Can you work these out from the model? Positions are in its coordinate system, mm. A direction names the side the tool comes from. Round coordinates to 2 decimals unless told otherwise and drop trailing zeros. Loops run counter-clockwise (first coordinate to the right, second up) from the corner with the lowest first, then second, coordinate; pieces in that order, holes last. Notation, with made-up numbers: (-12.5, 77) - (3.5, 77) arc R27 ccw to (3.5, 94) - close; hole circle Ø10 at (-15, -30). An arc over 180 degrees is marked (long way). Answer as CSV lines item,"result".
```python
from build123d import *

# Parameters (mm, degrees)
SKETCH_1_W          = 28.5
SKETCH_1_H          = 28.5
SKETCH_1_W_2        = 24.5
SKETCH_1_H_2        = 24.5
EXTRUDE_1_DEPTH     = 4
CUT_EXTRUDE_1_REACH = 34.114
SKETCH_2_W          = 15
SKETCH_2_H          = 4
EXTRUDE_2_DEPTH     = 1
SKETCH_4_W          = 2
SKETCH_4_H          = 5
EXTRUDE_3_DEPTH     = 7
EXTRUDE_7_DEPTH     = 5
SKETCH_6_W          = 6.5
SKETCH_6_H          = 6
SKETCH_6_R          = 1.75
EXTRUDE_6_DEPTH     = 2
FILLET_1_R          = 2
SKETCH_8_W          = 3
SKETCH_8_H          = 7.25
CUT_EXTRUDE_3_DEPTH = 40.358131307
FILLET_2_R          = 1


with BuildPart() as part:
    # ｽｹｯﾁ1 → ﾎﾞｽ - 押し出し1 (new body)
    with BuildSketch(Plane.XY):
        Rectangle(SKETCH_1_W, SKETCH_1_H)
        Rectangle(SKETCH_1_W_2, SKETCH_1_H_2, mode=Mode.SUBTRACT)
    extrude(amount=EXTRUDE_1_DEPTH)

    # ｽｹｯﾁ2 → ｶｯﾄ - 押し出し1 (cut, up to next)
    with BuildSketch(Plane(origin=(0, -14.25, 0), x_dir=(-1, 0, 0), z_dir=(0, -1, 0)), mode=Mode.PRIVATE) as cut_extrude_1_sk1:
        with Locations((0, -2)):
            Rectangle(SKETCH_2_W, SKETCH_2_H)
    cut_extrude_1_tool1 = extrude(cut_extrude_1_sk1.sketch, amount=-CUT_EXTRUDE_1_REACH, mode=Mode.PRIVATE) & part.part
    add(cut_extrude_1_tool1.solids().sort_by_distance((0, -14.25, 2))[0], mode=Mode.SUBTRACT)

    # ｽｹｯﾁ3 → ﾎﾞｽ - 押し出し2 (add)
    with BuildSketch(Plane(origin=(0, 0, 0), x_dir=(-1, 0, 0), z_dir=(0, 0, -1))):
        Polygon((12.25, 12.25), (12.25, -12.25), (7.5, -12.25), (7.5, -14.25), (14.25, -14.25), (14.25, 14.25), (-14.25, 14.25), (-14.25, -14.25), (-7.5, -14.25), (-7.5, -12.25), (-12.25, -12.25), (-12.25, 12.25), align=None)
        with BuildLine():
            Line((12.25, -12.25), (12.25, -10.25))
            ThreePointArc((12.25, -10.25), (11.664213562, -11.664213562), (10.25, -12.25))
            Line((10.25, -12.25), (12.25, -12.25))
        make_face()
        with BuildLine():
            Line((-7.5, -12.25), (-7.5, -11.25))
            Line((-7.5, -11.25), (-10.25, -11.25))
            ThreePointArc((-10.25, -11.25), (-10.957106781, -10.957106781), (-11.25, -10.25))
            Line((-11.25, -10.25), (-11.25, 10.25))
            ThreePointArc((-11.25, 10.25), (-10.957106781, 10.957106781), (-10.25, 11.25))
            Line((-10.25, 11.25), (10.25, 11.25))
            ThreePointArc((10.25, 11.25), (10.957106781, 10.957106781), (11.25, 10.25))
            Line((11.25, 10.25), (11.25, -10.25))
            ThreePointArc((11.25, -10.25), (10.957106781, -10.957106781), (10.25, -11.25))
            Line((10.25, -11.25), (7.5, -11.25))
            Line((7.5, -11.25), (7.5, -12.25))
            Line((7.5, -12.25), (10.25, -12.25))
            ThreePointArc((10.25, -12.25), (11.664213562, -11.664213562), (12.25, -10.25))
            Line((12.25, -10.25), (12.25, 10.25))
            ThreePointArc((12.25, 10.25), (11.664213562, 11.664213562), (10.25, 12.25))
            Line((10.25, 12.25), (-10.25, 12.25))
            ThreePointArc((-10.25, 12.25), (-11.664213562, 11.664213562), (-12.25, 10.25))
            Line((-12.25, 10.25), (-12.25, -10.25))
            ThreePointArc((-12.25, -10.25), (-11.664213562, -11.664213562), (-10.25, -12.25))
            Line((-10.25, -12.25), (-7.5, -12.25))
        make_face()
        with BuildLine():
            Line((-12.25, -12.25), (-10.25, -12.25))
            ThreePointArc((-10.25, -12.25), (-11.664213562, -11.664213562), (-12.25, -10.25))
            Line((-12.25, -10.25), (-12.25, -12.25))
        make_face()
        with BuildLine():
            Line((-12.25, 12.25), (-12.25, 10.25))
            ThreePointArc((-12.25, 10.25), (-11.664213562, 11.664213562), (-10.25, 12.25))
            Line((-10.25, 12.25), (-12.25, 12.25))
        make_face()
        with BuildLine():
            Line((12.25, 12.25), (10.25, 12.25))
            ThreePointArc((10.25, 12.25), (11.664213562, 11.664213562), (12.25, 10.25))
            Line((12.25, 10.25), (12.25, 12.25))
        make_face()
    extrude(amount=EXTRUDE_2_DEPTH)

    # ｽｹｯﾁ4 → ﾎﾞｽ - 押し出し3 (add)
    with BuildSketch(Plane.XY.offset(4)):
        with Locations((13.25, -2.5)):
            Rectangle(SKETCH_4_W, SKETCH_4_H)
        with Locations((-13.25, -2.5)):
            Rectangle(SKETCH_4_W, SKETCH_4_H)
    extrude(amount=EXTRUDE_3_DEPTH)

    # ｽｹｯﾁ5 → ﾎﾞｽ - 押し出し7 (add)
    with BuildSketch(Plane(origin=(0, 0, 0), x_dir=(1, 0, 0), z_dir=(0, 1, 0))):
        Polygon((12.25, -11), (11.5, -10), (12.25, -10), align=None)
        Polygon((-12.25, -11), (-11.5, -10), (-12.25, -10), align=None)
    extrude(amount=-EXTRUDE_7_DEPTH)

    # ｽｹｯﾁ6 → ﾎﾞｽ - 押し出し6 (add)
    # profile 1 of 2: a face of its own
    with BuildSketch(Plane(origin=(0, 0, -1), x_dir=(-1, 0, 0), z_dir=(0, 0, -1))):
        with Locations((17.5, -3)):
            Rectangle(SKETCH_6_W, SKETCH_6_H)
        with Locations((17.5, -3)):
            Circle(SKETCH_6_R, mode=Mode.SUBTRACT)
    # profile 2 of 2: a face of its own
    with BuildSketch(Plane(origin=(0, 0, -1), x_dir=(-1, 0, 0), z_dir=(0, 0, -1))):
        with Locations((-17.5, -3)):
            Rectangle(SKETCH_6_W, SKETCH_6_H)
        with Locations((-17.5, -3)):
            Circle(SKETCH_6_R, mode=Mode.SUBTRACT)
    extrude(amount=-EXTRUDE_6_DEPTH)

    # ﾌｨﾚｯﾄ1
    fillet_1_edges = [part.edges().sort_by_distance(p)[0] for p in [
        (20.75, -6, 0),
        (20.75, 0, 0),
        (-20.75, 0, 0),
        (-20.75, -6, 0),
        (14.25, 14.25, 1.5),
        (14.25, -14.25, 1.5),
        (-14.25, -14.25, 1.5),
        (-14.25, 14.25, 1.5),
    ]]
    fillet(fillet_1_edges, radius=FILLET_1_R)

    # ｽｹｯﾁ8 → ｶｯﾄ - 押し出し3 (cut, through all)
    with BuildSketch(Plane.ZY.offset(14.25)):
        with Locations((2.5, 3.625)):
            Rectangle(SKETCH_8_W, SKETCH_8_H)
    extrude(amount=-CUT_EXTRUDE_3_DEPTH, mode=Mode.SUBTRACT)

    # ﾌｨﾚｯﾄ2
    # the kernel refuses this fillet: 1 mm, written as the material it adds along each edge
    with BuildSketch(Plane(origin=(12.25, 7.25, 1), x_dir=(0, -1, 0), z_dir=(1, 0, 0))) as fillet_2_piece_1:
        with BuildLine():
            CenterArc((FILLET_2_R, -FILLET_2_R), FILLET_2_R, 90, 90)
            Line((0, -FILLET_2_R), (0, 0))
            Line((0, 0), (FILLET_2_R, 0))
        make_face()
    extrude(amount=2)
    with BuildSketch(Plane(origin=(12.25, 0, 1), x_dir=(0, 1, 0), z_dir=(1, 0, 0)), Plane(origin=(-14.25, 0, 1), x_dir=(0, 1, 0), z_dir=(1, 0, 0)), Plane(origin=(-14.25, 7.25, 1), x_dir=(0, 0, 1), z_dir=(1, 0, 0))) as fillet_2_piece_2:
        with BuildLine():
            CenterArc((FILLET_2_R, FILLET_2_R), FILLET_2_R, 180, 90)
            Line((0, FILLET_2_R), (0, 0))
            Line((0, 0), (FILLET_2_R, 0))
        make_face()
    extrude(amount=2)
    # the kernel refuses this fillet: 1 mm, written as the material it takes off along each edge
    with BuildSketch(Plane(origin=(9.75, 7.25, 4), x_dir=(0, 1, 0), z_dir=(1, 0, 0)), Plane(origin=(-16.75, 7.25, 4), x_dir=(0, 1, 0), z_dir=(1, 0, 0))) as fillet_2_2_piece_1:
        with BuildLine():
            CenterArc((FILLET_2_R, -FILLET_2_R), FILLET_2_R, 90, 90)
            Line((0, -FILLET_2_R), (0, 0))
            Line((0, 0), (FILLET_2_R, 0))
        make_face()
    extrude(amount=7, mode=Mode.SUBTRACT)


solid = part.part
```
Q1. Imagine slicing it at B-B (y = -3). Write out the boundary of the cut face in (x, z).
Checks:
outline,"(-20.75, -1) - (-19.25, -1) - (-19.25, 1) - (-20.75, 1) - close; (-15.75, -1) - (-11.25, -1) - (-11.25, 0) - (-12.25, 0) - (-12.25, 10) - (-11.5, 10) - (-12.25, 11) - (-14.25, 11) - (-14.25, 1) - (-15.75, 1) - close; (11.25, -1) - (15.75, -1) - (15.75, 1) - (14.25, 1) - (14.25, 11) - (12.25, 11) - (11.5, 10) - (12.25, 10) - (12.25, 0) - (11.25, 0) - close; (19.25, -1) - (20.75, -1) - (20.75, 1) - (19.25, 1) - close"
Q2. Imagine slicing it at A-A (z = 5.5). Write out the boundary of the cut face in (x, y), then the cut area to 3 significant figures.
Checks:
outline,"(-14.25, -5) - (-12.25, -5) - (-12.25, 0) - (-14.25, 0) - close; (12.25, -5) - (14.25, -5) - (14.25, 0) - (12.25, 0) - close"
area,"20.0 mm²"
Q3. On a 3-axis mill with a long thin cutter (end or side, diameter ignored), from which of +Z, -Z, +X, -X, +Y, -Y can I reach the whole of each face in a straight line? I mean faces 4 (the flat face through (-11.25, 0.1, -0.5)), 5 (the flat face through (0, 12.25, 2)), 6 (the flat face through (-13, 0, 6)). Say none if no direction works.
Checks:
face 4,"+Z, -Z"
face 5,"+Z"
face 6,"+Z, +X, -X"
Q4. Imagine slicing it at C-C (x = -17.5). Write out the boundary of the cut face in (y, z), then the cut area to 3 significant figures.
Checks:
outline,"(-6, -1) - (-4.75, -1) - (-4.75, 1) - (-6, 1) - close; (-1.25, -1) - (0, -1) - (0, 1) - (-1.25, 1) - close"
area,"5.00 mm²"
Q5. If I drill on line 1 along Y through (x, z) = (-17.5, -0.55); line 2 along X through (y, z) = (-0.5, 6.75); line 3 along Y through (x, z) = (-6, 0.75), over which ranges is the centre line in solid material (lowest first)? Write a range as [from, to].
Checks:
line 1,"[-6, -4.75], [-1.25, 0]"
line 2,"[-14.25, -12.25], [12.25, 14.25]"
line 3,"[12.25, 14.25]"
Q6. Imagine slicing it at D-D (x = -4.5). Write out the boundary of the cut face in (y, z).
Checks:
outline,"(11.25, -1) - (14.25, -1) - (14.25, 4) - (12.25, 4) - (12.25, 0) - (11.25, 0) - close"
Q7. I'm going to push flat-ended pins straight in: pin 1 Ø1.5 at (x, y) = (14, -7) entering from +Z; pin 2 Ø1 at (x, y) = (-13.5, 4.5) entering from +Z; pin 3 Ø1.4 at (x, z) = (13, 6.5) entering from +Y. Where does each tip first touch, or does it pass through?
Checks:
pin 1,"z = 4"
pin 2,"z = 1"
pin 3,"y = 0"
Q8. We'd pull the mould along X, two halves only. Please class faces 1 (the flat face through (-10, -12.25, 2)), 2 (the cylindrical face through (-13.65, 13.68, 1.46)), 3 (the flat face through (13, -2, 11)): pulls with the +X half, pulls with the -X half, needs draft (parallel to the pull), parting line crosses it, or undercut.
Checks:
face 1,"undercut"
face 2,"pulls with the -X half"
face 3,"needs draft"
